For this review, take the finished solid that the model builds, in its own axes (mm). A direction names the side the tool comes from. Coordinates: 2 decimals unless noted, no trailing zeros. Loops run counter-clockwise (first coordinate to the right, second up) from the corner with the lowest first, then second, coordinate; pieces in that order, holes last. Notation, with made-up numbers: M -27.5,42.25 L 31.5,42.25 A22 cw 31.5,78.25 Z; hole C 70,47 d11. An arc over 180 degrees is marked long. Answer as a JSON object with one key per item and string values. Group by question number.
Item 1: Add section B-B (x = 82.55). State the section outline as (y, z) points (3 decimals).
Item 2: Wall thickness on L1, parallel to X at y = 1.4, z = -12.7 (3 decimals); L2, parallel to X at y = 0.65, z = -11 (3 decimals); L3, parallel to Z at x = 29.5, y = 0.65: over which ranges is each line inside the solid? List them lowest first. Write a range as from..to.
Item 3: Tool access review of faces 1 (the face through (16.83, 1.565, -7.255)), 2 (the face through (48, 2, -25.4)): name each direction out of +Z, -Z, +X, -X, +Y, -Y from which nothing blocks a thin tool from reaching the whole face with its end or side.
Item 4: Add section C-C (y = 2.45). State the section outline as (x, z) points (3 decimals).
Item 5: Add section A-A (z = -12.7). State the section outline as (x, y) points (3 decimals), then the cut area to 3 significant figures.
Item 6: Mouldability with a two-part tool opening along X and no side actions: class faces 3 (the face through (0, 2, -13)), 4 (the face through (95.25, 2, -13)), 5 (the face through (16.78, 1.565, -18.095)), 6 (the face through (47, 3.175, -13)) as +X half, -X half, draft (parallel to the pull), parting line (faces both ways), or undercut.
from build123d import *

# Parameters (mm, degrees)
SKETCH1_R           = 3.175
BOSS_EXTRUDE1_DEPTH = 3.175


with BuildPart() as part:
    # Sketch1 → Boss-Extrude1 (new body)
    with BuildSketch(Plane(origin=(0, 0, 0), x_dir=(1, 0, 0), z_dir=(0, 1, 0))):
        Polygon((0, 4.7625), (0, 0), (6.35, 0), (44.45, 0), (57.15, 0), (95.25, 0), (95.25, 25.4), (57.15, 25.4), (44.45, 25.4), (6.35, 25.4), (0, 25.4), (0, 20.6375), align=None)
        with Locations(Location((82.55, 12.7, 0), (0, 0, 270))):
            Circle(SKETCH1_R, mode=Mode.SUBTRACT)
        with BuildLine():
            ThreePointArc((15.875, 15.875), (16.80493597, 18.12006403), (19.05, 19.05))
            Line((19.05, 19.05), (31.75, 19.05))
            ThreePointArc((31.75, 19.05), (33.99506403, 18.12006403), (34.925, 15.875))
            Line((34.925, 15.875), (34.925, 9.525))
            ThreePointArc((34.925, 9.525), (33.99506403, 7.27993597), (31.75, 6.35))
            Line((31.75, 6.35), (19.05, 6.35))
            ThreePointArc((19.05, 6.35), (16.80493597, 7.27993597), (15.875, 9.525))
            Line((15.875, 9.525), (15.875, 15.875))
        make_face(mode=Mode.SUBTRACT)
    extrude(amount=BOSS_EXTRUDE1_DEPTH)


solid = part.part
From the geometry:
{
 "1": {"outline": "M 0,-25.4 L 3.175,-25.4 L 3.175,-15.875 L 0,-15.875 Z; M 0,-9.525 L 3.175,-9.525 L 3.175,0 L 0,0 Z"},
 "2": {"L1": "x = 0..15.875, 34.925..79.375, 85.725..95.25", "L2": "x = 0..15.875, 34.925..79.868, 85.232..95.25", "L3": "z = -25.4..-19.05, -6.35..0"},
 "3": {"face 1": "+Y, -Y", "face 2": "-Z, +X, -X, +Y, -Y"},
 "4": {"outline": "M 0,-25.4 L 95.25,-25.4 L 95.25,0 L 0,0 Z; hole M 15.875,-15.875 A3.175 ccw 19.05,-19.05 L 31.75,-19.05 A3.175 ccw 34.925,-15.875 L 34.925,-9.525 A3.175 ccw 31.75,-6.35 L 19.05,-6.35 A3.175 ccw 15.875,-9.525 Z; hole C 82.55,-12.7 d6.35"},
 "5": {"outline": "M 0,0 L 15.875,0 L 15.875,3.175 L 0,3.175 Z; M 34.925,0 L 79.375,0 L 79.375,3.175 L 34.925,3.175 Z; M 85.725,0 L 95.25,0 L 95.25,3.175 L 85.725,3.175 Z", "area": "222 mm²"},
 "6": {"face 3": "-X half", "face 4": "+X half", "face 5": "undercut", "face 6": "draft"}
}
